from build123d import *

# Parameters (mm, degrees)
F0_R     = 2
F1_DEPTH = 7
F3_DEPTH = 5.25
F4_DEPTH = 1.75
F5_R     = 2
F6_DEPTH = 1.75


with BuildPart() as f1:
    # F0 (on Top) → F1 (new body)
    with BuildSketch(Plane.XY):
        with BuildLine():
            Line((40.009908, 0), (5.040038, 0))
            ThreePointArc((5.040038, 0), (0.664349, -7.419369), (9.274601, -7.658661))
            Line((9.274601, -7.658661), (15.540038, -8.6))
            Line((15.540038, -8.6), (36.540038, -8.6))
            ThreePointArc((36.540038, -8.6), (41.176847, -5.470829), (40.009908, 0))
        make_face()
        with Locations((5.040038, -5)):
            Circle(F0_R, mode=Mode.SUBTRACT)
        with Locations((36.540038, -3.6)):
            Circle(F0_R, mode=Mode.SUBTRACT)
    extrude(amount=F1_DEPTH)

    # F2 (on face) → F3 (cut)
    with BuildSketch(Plane.XY.offset(7)):
        with BuildLine():
            Line((11.540038, 0), (5.040038, 0))
            ThreePointArc((5.040038, 0), (2.831279, -9.485687), (9.003158, -1.951446))
            Line((9.003158, -1.951446), (11.540038, 0))
        make_face()
    extrude(amount=-F3_DEPTH, mode=Mode.SUBTRACT)

    # F2 (on face) → F4 (join)
    with BuildSketch(Plane.XY.offset(7)):
        with BuildLine():
            Line((11.540038, 0), (5.040038, 0))
            ThreePointArc((5.040038, 0), (2.831279, -9.485687), (9.003158, -1.951446))
            Line((9.003158, -1.951446), (11.540038, 0))
        make_face()
    extrude(amount=-F4_DEPTH)

    # F5 (on face) → F6 (cut)
    with BuildSketch(Plane.XY.offset(7)):
        with Locations((5.040038, -5)):
            Circle(F5_R)
    extrude(amount=-F6_DEPTH, mode=Mode.SUBTRACT)


solid = f1.part
Geometry: final body of the model. Coordinates: model frame, mm. A direction names the side the tool comes from. Give positions to 0.01 mm unless a question says otherwise; leave off trailing zeros. Order: outer loops, then holes, each group sorted by start corner. A loop starts at its lowest first (then second) coordinate and runs counter-clockwise, first axis right, second up. Notation, with made-up numbers: (-24.75, 46) -> (32.25, 46) arc R18 cw to (32.25, 59) -> close; hole circle Ø4 at (72, 4.5). An arc over 180 degrees is marked (long way). Answer as a JSON object with one key per item and string values.
Q1. Section A-A (z = 3). Output: boundary loops of the cut face in (x, y), plus the area to 3 significant figures.
Entries:
{"outline": "(9, -1.95) arc R5 cw to (9.27, -7.66) -> (15.54, -8.6) -> (36.54, -8.6) arc R5 ccw to (40.01, 0) -> (11.54, 0) -> close; hole circle Ø4 at (36.54, -3.6)", "area": "250 mm^2"}
Q2. Draft query along Y for faces 5 (the cylindrical face through (5, -7, 1)), 6 (the flat face through (20, -4, 0)), 7 (the flat face through (10.25, -0.99, 3.52)). Return one class per face: released by +Y, released by -Y, zero draft, split by the parting line, or undercut.
Entries:
{"face 5": "undercut", "face 6": "zero draft", "face 7": "released by +Y"}
Q3. Section C-C (y = -5). Output: boundary loops of the cut face in (x, z).
Entries:
{"outline": "(0.04, 0) -> (3.04, 0) -> (3.04, 1.75) -> (0.04, 1.75) -> close; (0.04, 5.25) -> (3.04, 5.25) -> (3.04, 7) -> (0.04, 7) -> close; (7.04, 0) -> (35.11, 0) -> (35.11, 7) -> (7.04, 7) -> (7.04, 5.25) -> (10.04, 5.25) -> (10.04, 1.75) -> (7.04, 1.75) -> close; (37.97, 0) -> (41.34, 0) -> (41.34, 7) -> (37.97, 7) -> close"}
Q4. Material intervals for probe 1 along Z at (x, y) = (8, -4.5); probe 2 along X at (y, z) = (-5, 1); probe 3 along Y at (x, z) = (32.5, 2), sorted ascending.
Entries:
{"probe 1": "z = 0 to 1.75, 5.25 to 7", "probe 2": "x = 0.04 to 3.04, 7.04 to 35.11, 37.97 to 41.34", "probe 3": "y = -8.6 to 0"}
Q5. Section B-B (z = 5.75). Output: boundary loops of the cut face in (x, y).
Entries:
{"outline": "(5.04, 0) arc R5 ccw (long way) to (9.27, -7.66) -> (15.54, -8.6) -> (36.54, -8.6) arc R5 ccw to (40.01, 0) -> close; hole circle Ø4 at (5.04, -5); hole circle Ø4 at (36.54, -3.6)"}
Q6. Access query for faces 1 (the flat face through (26, -8.6, 3)), 2 (the cylindrical face through (10.036, -4.805, 3.524)), 3 (the flat face through (12.363, -8.123, 3.451)), 4 (the flat face through (23, 0, 4)). Directions: +Z, -Z, +X, -X, +Y, -Y. A direction counts if a zero-diameter tool reaches every point of the face in a straight line with its end or side. Return the directions, or none.
Entries:
{"face 1": "+Z, -Z, +X, -Y", "face 2": "-X", "face 3": "+Z, -Z, -Y", "face 4": "+Z, -Z, +X, -X, +Y"}
Q7. Section D-D (y = -8.25). Output: boundary loops of the cut face in (x, z), plus the area to 3 significant figures.
Entries:
{"outline": "(1.24, 0) -> (8.84, 0) -> (8.84, 1.75) -> (1.24, 1.75) -> close; (1.24, 5.25) -> (8.84, 5.25) -> (8.84, 7) -> (1.24, 7) -> close; (13.21, 0) -> (38.38, 0) -> (38.38, 7) -> (13.21, 7) -> close", "area": "203 mm^2"}
